Source: CAD feature listing. Evaluate the final solid. Frame: model axes, mm. A direction names the side the tool comes from. Round coordinates to 2 decimals unless told otherwise and drop trailing zeros. Write each loop counter-clockwise with the first axis right and the second up, starting at its lowest first coordinate (ties: lowest second). Pieces come first, ordered by that corner, then holes. Notation, with made-up numbers: M 83,17 L 97,17 A30 ccw 97,43 Z; hole C 81,-20.5 d1. An arc over 180 degrees is marked long. Answer in a Markdown table with one row per item. Add a question column.
Item 1: Cut plane D-D on z = -82. Return loops of the section in (x, y), and give its area (3 significant figures).
Item 2: Cut plane A-A on z = -38.5. Return loops of the section in (x, y).
Item 3: Mould query, pull axis X, two halves, no side actions, for faces 1 (the face through (12, 7, -46)), 2 (the face through (0, 28, -46)), 3 (the face through (23.5, 31, -39)). Classes: released by +X, released by -X, zero draft, split by the parting line, or undercut.
Item 4: Material intervals for probe 1 along Z at (x, y) = (4.5, 3); probe 2 along Y at (x, z) = (12, -86); probe 3 along Y at (x, z) = (20, -54.5), sorted ascending.
Item 5: Cut plane C-C on y = 31. Return loops of the section in (x, z), and give its area (3 significant figures).
Item 6: Cut plane B-B on z = -29. Return loops of the section in (x, y).
Item 7: Set-up query: faces 4 (the face through (12, 4, -42)), 5 (the face through (14.419, 20.794, -5.916)), 6 (the face through (12, 27, -45)). Return all of +Z, -Z, +X, -X, +Y, -Y with unobstructed straight access to the full face (end or side cutting, diameter ignored); none if empty.
Autodesk Inventor part; units mm, degrees
ref_plane "YZ Plane" through (0, 0, 0) normal (1, 0, 0) x (0, 1, 0)
ref_plane "XZ Plane" through (0, 0, 0) normal (0, 1, 0) x (-1, 0, 0)
ref_plane "XY Plane" through (0, 0, 0) normal (0, 0, 1) x (1, 0, 0)
sketch "Sketch1" plane through (0, 0, 0) normal (0, 1, 0) x (-1, 0, 0)
  line L0 (0, 0) -> (-24, 0)
  line L1 (-24, 0) -> (-24, -91)
  line L2 (-24, -91) -> (0, -91)
  line L3 (0, -91) -> (0, 0)
  dimension "d0" = 91
  dimension "d1" = 24
extrude "Extrusion1" add sketch "Sketch1" along normal blind 34
sketch "Sketch2" plane through (24, 0, 0) normal (1, 0, 0) x (0, 0, -1)
  line L0 (22, 27) -> (69, 27)
  line L1 (69, 27) -> (69, 7)
  line L2 (69, 7) -> (22, 7)
  line L3 (22, 7) -> (22, 27)
  line L4 (0, 34) -> (91, 34)
  line L5 (0, 0) -> (91, 0)
  line L6 (0, 0) -> (0, 34)
  line L7 (91, 0) -> (91, 34)
  dimension "d4" = 7
  dimension "d5" = 7
  dimension "d6" = 22
  dimension "d7" = 22
extrude "Extrusion2" cut sketch "Sketch2" against normal up to surface (24 mm away) contours L0 L1 L2 L3
sketch "Sketch3" plane through (0, 34, 0) normal (0, 1, 0) x (1, 0, 0)
  line L0 (0.5, 42) -> (23.5, 42)
  line L1 (23.5, 42) -> (23.5, 36)
  line L2 (23.5, 36) -> (0.5, 36)
  line L3 (0.5, 36) -> (0.5, 42)
  line L4 (0, 91) -> (0, 0)
  line L5 (24, 0) -> (24, 91)
  line L6 (0, 0) -> (24, 0)
  dimension "d10" = 0.5
  dimension "d11" = 0.5
  dimension "d12" = 6
  dimension "d13" = 36
extrude "Extrusion3" cut sketch "Sketch3" against normal up to surface (34 mm away)
sketch "Sketch4" plane through (0, 34, 0) normal (0, 1, 0) x (1, 0, 0)
  line L0 (0.5, 51) -> (23.5, 51)
  line L1 (23.5, 51) -> (23.5, 49)
  line L2 (23.5, 49) -> (0.5, 49)
  line L3 (0.5, 49) -> (0.5, 51)
  line L4 (0.5, 42) -> (23.5, 42)
  line L5 (24, 0) -> (24, 91)
  line L6 (0, 91) -> (0, 0)
  dimension "d16" = 2
  dimension "d17" = 7
  dimension "d18" = 0.5
  dimension "d19" = 0.5
extrude "Extrusion4" cut sketch "Sketch4" against normal up to surface (34 mm away)
sketch "Sketch5" plane through (0, 0, 0) normal (0, 0, 1) x (1, 0, 0)
  circle A0 centre (12, 17) radius 4.5
  line L0 (0, 0) -> (24, 0)
  line L1 (24, 0) -> (24, 34)
  dimension "d22" = 17
  dimension "d23" = 12
  dimension "d24" = 9
extrude "Extrusion5" cut sketch "Sketch5" against normal blind 12
loft "Loft1" cut section 1 edges at (7.5, 17, -12) section 2 edges at (0, 17, -22) (12, 27, -22) (24, 17, -22) (12, 7, -22)
sketch "Sketch6" plane through (24, 0, -91) normal (0, 0, -1) x (-1, 0, 0)
  circle A0 centre (12, 17) radius 4.5
  line L0 (24, 0) -> (24, 34)
  line L1 (0, 0) -> (24, 0)
  dimension "d31" = 12
  dimension "d32" = 17
  dimension "d33" = 9
extrude "Extrusion6" cut sketch "Sketch6" against normal blind 12
loft "Loft2" cut section 1 edges at (16.5, 17, -79) section 2 edges at (0, 17, -69) (12, 7, -69) (24, 17, -69) (12, 27, -69)
properties part number "20220727_1cell_PBME"
Results below:
| question | item | result |
|---|---|---|
| 1 | outline | M 0,0 L 24,0 L 24,34 L 0,34 Z; hole C 12,17 d9 |
| 1 | area | 752 mm2 |
| 2 | outline | M 0,0 L 0.5,0 L 0.5,7 L 0,7 Z; M 0,27 L 0.5,27 L 0.5,34 L 0,34 Z; M 23.5,0 L 24,0 L 24,7 L 23.5,7 Z; M 23.5,27 L 24,27 L 24,34 L 23.5,34 Z |
| 3 | face 1 | zero draft |
| 3 | face 2 | released by -X |
| 3 | face 3 | undercut |
| 4 | probe 1 | -91 to -51, -49 to -42, -36 to 0 |
| 4 | probe 2 | 0 to 12.5, 21.5 to 34 |
| 4 | probe 3 | 0 to 7, 27 to 34 |
| 5 | outline | M 0,-91 L 24,-91 L 24,0 L 0,0 Z; hole M 0.5,-51 L 23.5,-51 L 23.5,-49 L 0.5,-49 Z; hole M 0.5,-42 L 23.5,-42 L 23.5,-36 L 0.5,-36 Z |
| 5 | area | 2,000 mm2 |
| 6 | outline | M 0,0 L 24,0 L 24,7 L 0,7 Z; M 0,27 L 24,27 L 24,34 L 0,34 Z |
| 7 | face 4 | +Y, -Y |
| 7 | face 5 | +Z, -Z |
| 7 | face 6 | +X, -X |
